from build123d import *

# Parameters (mm, degrees)
CROQUIS1_R              = 12.5
SALIENTE_EXTRUIR1_DEPTH = 50
CROQUIS3_R              = 1.25
CROQUIS3_R_2            = 3
CORTAR_EXTRUIR1_DEPTH   = 51
CROQUIS6_R              = 1.5
CORTAR_EXTRUIR2_DEPTH   = 26


with BuildPart() as part:
    # Croquis1 → Saliente-Extruir1 (new body)
    with BuildSketch(Plane.XY):
        Circle(CROQUIS1_R)
    extrude(amount=SALIENTE_EXTRUIR1_DEPTH)

    # Croquis3 → Cortar-Extruir1 (cut, through all)
    with BuildSketch(Plane.XY.offset(50)):
        with Locations((8.75, 0)):
            Circle(CROQUIS3_R)
        with Locations((4.375, -7.577722283)):
            Circle(CROQUIS3_R)
        with Locations((-4.375, -7.577722283)):
            Circle(CROQUIS3_R)
        with Locations((-8.75, 0)):
            Circle(CROQUIS3_R)
        with Locations((-4.375, 7.577722283)):
            Circle(CROQUIS3_R)
        with Locations((4.375, 7.577722283)):
            Circle(CROQUIS3_R)
        Circle(CROQUIS3_R_2)
    extrude(amount=-CORTAR_EXTRUIR1_DEPTH, mode=Mode.SUBTRACT)

    # Croquis6 → Cortar-Extruir2 (cut, through all)
    with BuildSketch(Plane(origin=(0, 12.5, 0), x_dir=(1, 0, 0), z_dir=(0, 1, 0))):
        with Locations((0, -5)):
            Circle(CROQUIS6_R)
    extrude(amount=-CORTAR_EXTRUIR2_DEPTH, mode=Mode.SUBTRACT)


solid = part.part
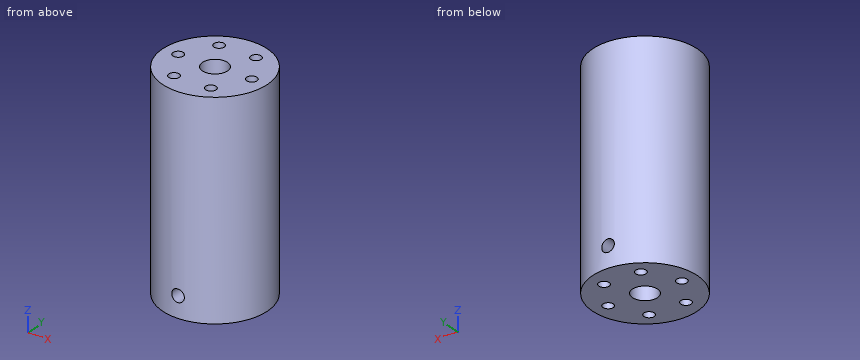
The listing builds one solid part. Answer for the finished solid, in the listing's coordinates (mm). Give positions to 0.01 mm unless a question says otherwise; leave off trailing zeros. Loops run counter-clockwise (first coordinate to the right, second up) from the corner with the lowest first, then second, coordinate; pieces in that order, holes last.
Item 1: A cutting plane is placed at A-A (y = 0). Give the vertices of the cut face in (x, z), then the cut area to 3 significant figures.
Derived:
outline: (-12.5, 0) - (-10, 0) - (-10, 50) - (-12.5, 50) - close; (-7.5, 0) - (-3, 0) - (-3, 50) - (-7.5, 50) - close; (3, 0) - (7.5, 0) - (7.5, 50) - (3, 50) - close; (10, 0) - (12.5, 0) - (12.5, 50) - (10, 50) - close
area: 700 mm2
Item 2: Each of these flat-tipped pins is pushed along its axis until it touches: pin 1 Ø12 at (x, z) = (9, 18) entering from -Y; pin 2 Ø4 at (y, z) = (6.5, 15) entering from +X; pin 3 Ø1 at (y, z) = (-8, 24.5) entering from +X. Where does it stop, or does it pass through?
Derived:
pin 1: stops at y = -12.13
pin 2: stops at x = 11.66
pin 3: stops at x = 10
Item 3: Find the intervals of material crossed by line 1 along X through (y, z) = (-0.75, 18.5); line 2 along Z through (x, y) = (0, 10.25); line 3 along X through (y, z) = (7.25, 5), in increasing order.
Derived:
line 1: x = -12.48 to -9.75, -7.75 to -2.9, 2.9 to 7.75, 9.75 to 12.48
line 2: z = 0 to 3.5, 6.5 to 50
line 3: x = -10.18 to -5.58, -3.17 to -1.5, 1.5 to 3.17, 5.58 to 10.18
Item 4: A cutting plane is placed at C-C (x = -2.25). Give the vertices of the cut face in (y, z).
Derived:
outline: (-12.3, 0) - (-1.98, 0) - (-1.98, 50) - (-12.3, 50) - close; (1.98, 0) - (12.3, 0) - (12.3, 50) - (1.98, 50) - close
Item 5: A cutting plane is placed at B-B (z = 5). Give the vertices of the cut face in (x, y) (3 decimals).
Derived:
outline: (-1.5, -12.41) - (-1.5, -2.598) arc R3 cw to (-1.5, 2.598) - (-1.5, 12.41) arc R12.5 ccw to start; (1.5, -12.41) arc R12.5 ccw to (1.5, 12.41) - (1.5, 2.598) arc R3 cw to (1.5, -2.598) - close; hole circle Ø2.5 at (-8.75, 0); hole circle Ø2.5 at (-4.375, -7.578); hole circle Ø2.5 at (-4.375, 7.578); hole circle Ø2.5 at (4.375, -7.578); hole circle Ø2.5 at (4.375, 7.578); hole circle Ø2.5 at (8.75, 0)
Item 6: A cutting plane is placed at D-D (y = -3.5). Give the vertices of the cut face in (x, z).
Derived:
outline: (-12, 0) - (12, 0) - (12, 50) - (-12, 50) - close; hole circle Ø3 at (0, 5)
